The model under review builds one solid part; all positions refer to its coordinate system, in mm. Face numbers are marked on the shaded views. A direction names the side the tool comes from. Coordinates: 2 decimals unless noted, no trailing zeros. Loops run counter-clockwise (first coordinate to the right, second up) from the corner with the lowest first, then second, coordinate; pieces in that order, holes last. Notation, with made-up numbers: M 27.5,32.25 L 38.5,32.25 A25 ccw 38.5,48.25 Z; hole C 52.25,35 d7. An arc over 180 degrees is marked long. Return JSON: item names as keys, results as strings.
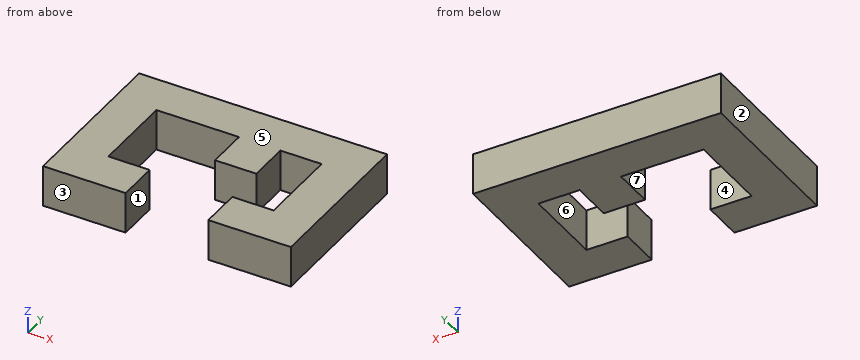
```python
from build123d import *

# Parameters (mm, degrees)
F0_W     = 10
F0_H     = 10
F1_DEPTH = 10


with BuildPart() as f1:
    # F0 (on Top) → F1 (new body)
    with BuildSketch(Plane.XY):
        Polygon((30, 20), (-30, 20), (-30, -20), (-10, -20), (-10, -10), (-20, -10), (-20, 10), (0, 10), (10, 10), (20, 10), (20, -10), (10, -10), (10, -20), (30, -20), align=None)
        with Locations((5, 5)):
            Rectangle(F0_W, F0_H)
    extrude(amount=F1_DEPTH)


solid = f1.part
```
1. The part is to be moulded in two halves that separate along X. For the marked faces 1, 2, 3 and 4, say which applies: released by +X, released by -X, zero draft, split by the parting line, or undercut.
Check values:
{"face 1": "undercut", "face 2": "released by -X", "face 3": "zero draft", "face 4": "undercut"}
2. Add section B-B on x = -17. Give the boundary of the cut face in (y, z), plus the area to 3 significant figures.
Check values:
{"outline": "M -20,0 L -10,0 L -10,10 L -20,10 Z; M 10,0 L 20,0 L 20,10 L 10,10 Z", "area": "200 mm²"}
3. Add section A-A on y = -13. Give the boundary of the cut face in (x, z).
Check values:
{"outline": "M -30,0 L -10,0 L -10,10 L -30,10 Z; M 10,0 L 30,0 L 30,10 L 10,10 Z"}
4. Add section C-C on y = 5. Give the boundary of the cut face in (x, z), plus the area to 3 significant figures.
Check values:
{"outline": "M -30,0 L -20,0 L -20,10 L -30,10 Z; M 0,0 L 10,0 L 10,10 L 0,10 Z; M 20,0 L 30,0 L 30,10 L 20,10 Z", "area": "300 mm²"}
5. Insertion check: pin 1 Ø5 at (x, z) = (5.5, 3) entering from -Y; pin 2 Ø12 at (x, y) = (-8.5, -9.5) entering from +Z. Each pin has a flat end and moves straight along its axis. Give the tip position at first contact, or say it passes through.
Check values:
{"pin 1": "y = 0", "pin 2": "z = 10"}
6. To check wall thickness, follow line 1 (X direction, y = 4, z = 7.75); line 2 (Y direction, x = -17.5, z = 2); line 3 (X direction, y = -13, z = 6.75). State the ranges of each line that lie inside material, in increasing order.
Check values:
{"line 1": "-30 to -20, 0 to 10, 20 to 30", "line 2": "-20 to -10, 10 to 20", "line 3": "-30 to -10, 10 to 30"}
7. Machinability: for the marked faces 5, 6 and 7, which of the approach directions +Z, -Z, +X, -X, +Y, -Y give a long, thin tool a straight path to every point of the face, cutting with its end or side? Answer none if there is none.
Check values:
{"face 5": "+Z, +X, -X, +Y, -Y", "face 6": "+Z, -Z", "face 7": "+Z, -Z, -Y"}
8. Add section D-D on z = 7.25. Give the boundary of the cut face in (x, y), plus the area to 3 significant figures.
Check values:
{"outline": "M -30,-20 L -10,-20 L -10,-10 L -20,-10 L -20,10 L 0,10 L 0,0 L 10,0 L 10,10 L 20,10 L 20,-10 L 10,-10 L 10,-20 L 30,-20 L 30,20 L -30,20 Z", "area": "1,500 mm²"}
